```python
from build123d import *

# Parameters (mm, degrees)
SKETCH1_W           = 350
SKETCH1_H           = 60
BOSS_EXTRUDE1_DEPTH = 15
SKETCH2_R           = 4
CUT_EXTRUDE1_DEPTH  = 356.422284051


with BuildPart() as part:
    # Sketch1 → Boss-Extrude1 (new body)
    with BuildSketch(Plane(origin=(0, 0, 0), x_dir=(1, 0, 0), z_dir=(0, 1, 0))):
        with Locations((175, -30)):
            Rectangle(SKETCH1_W, SKETCH1_H)
    extrude(amount=BOSS_EXTRUDE1_DEPTH)

    # Sketch2 → Cut-Extrude1 (cut, through all)
    with BuildSketch(Plane(origin=(0, 15, 0), x_dir=(1, 0, 0), z_dir=(0, 1, 0))):
        with Locations(Location((23, -48, 0), (0, 0, 270))):
            Circle(SKETCH2_R)
        with Locations(Location((61, -48, 0), (0, 0, 270))):
            Circle(SKETCH2_R)
        with Locations(Location((99, -48, 0), (0, 0, 270))):
            Circle(SKETCH2_R)
        with Locations(Location((137, -48, 0), (0, 0, 270))):
            Circle(SKETCH2_R)
        with Locations(Location((175, -48, 0), (0, 0, 270))):
            Circle(SKETCH2_R)
        with Locations(Location((213, -48, 0), (0, 0, 270))):
            Circle(SKETCH2_R)
        with Locations(Location((251, -48, 0), (0, 0, 270))):
            Circle(SKETCH2_R)
        with Locations(Location((289, -48, 0), (0, 0, 270))):
            Circle(SKETCH2_R)
        with Locations(Location((327, -48, 0), (0, 0, 270))):
            Circle(SKETCH2_R)
    extrude(amount=-CUT_EXTRUDE1_DEPTH, mode=Mode.SUBTRACT)


solid = part.part
```
Design review of the part built by this model. Coordinates are the model's own, in mm. Give positions to 0.01 mm unless a question says otherwise; leave off trailing zeros. Write each loop counter-clockwise with the first axis right and the second up, starting at its lowest first coordinate (ties: lowest second). Pieces come first, ordered by that corner, then holes.
(1) Mouldability with a two-part tool opening along X and no side actions: class faces 1 (the face through (173, 7, 60)), 2 (the face through (140.966, 7.605, 47.479)), 3 (the face through (350, 7, 30)), 4 (the face through (0, 7, 30)) as +X half, -X half, draft (parallel to the pull), parting line (faces both ways), or undercut.
Checked values:
face 1: draft
face 2: undercut
face 3: +X half
face 4: -X half
(2) Add section A-A (y = 9.5). Give the number of separate pieces and of enclosed holes in the cut face, and give its area (3 significant figures).
Checked values:
separate pieces: 1
enclosed holes: 9
area: 20,500 mm2
(3) Wall thickness on line 1 along Z through (x, y) = (289, 4.25); line 2 along Z through (x, y) = (328.5, 1.75): over which ranges is each line inside the solid? List them lowest first.
Checked values:
line 1: z = 0 to 44, 52 to 60
line 2: z = 0 to 44.29, 51.71 to 60
(4) Clearance check with a flat-ended pin moving along its axis: pin 1 Ø6.5 at (x, z) = (251, 48) entering from -Y. State where the tip first meets the part, or that it passes through.
Checked values:
pin 1: passes through
(5) Add section B-B (x = 289). Give the boundary of the cut face in (y, z), and give its area (3 significant figures).
Checked values:
outline: (0, 0) - (15, 0) - (15, 44) - (0, 44) - close; (0, 52) - (15, 52) - (15, 60) - (0, 60) - close
area: 780 mm2
